Here's the drawing with two shaded views (mm, measured from the low corner). I have some questions. A direction names the side the tool comes from. Round coordinates to 2 decimals unless told otherwise and drop trailing zeros. Return JSON: item names as keys, results as strings. Group by question number.
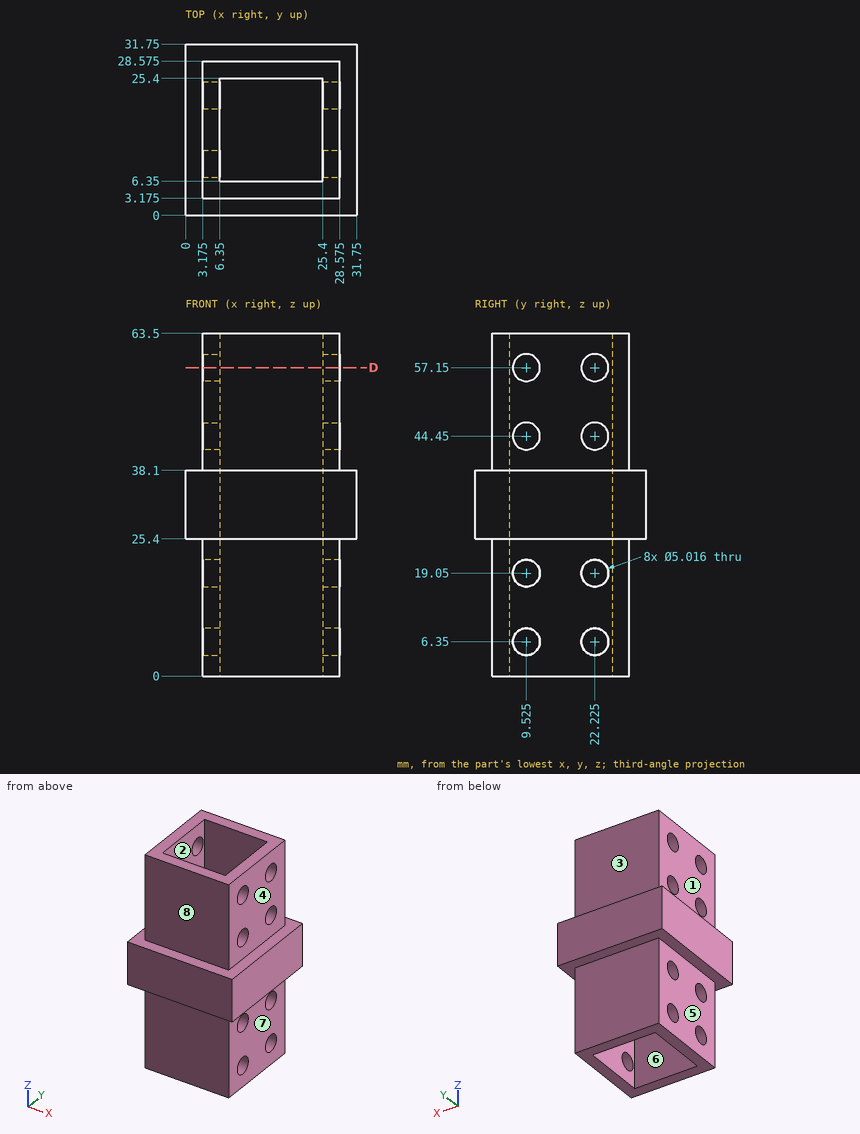
1) We'd pull the mould along X, two halves only. Please class the marked faces 1, 2 and 3: +X half, -X half, draft (parallel to the pull), parting line (faces both ways), or undercut.
2) Will these pins go through, and if not, where does the flat tip stop? pin 1 (1.5 mm diameter, centred on x = 11, z = 18, fed in from -Y) (1 decimal); pin 2 (6 mm diameter, centred on y = 9.525, z = 44.45, fed in from -X) (1 decimal); pin 3 (6.5 mm diameter, centred on y = 22.225, z = 44.45, fed in from +X) (1 decimal).
3) I want a section at D-D, the plane z = 57.15. Give the number of separate pieces and of enclosed holes in the cut face.
4) For the marked faces 4, 5, 6, 7 and 8, which set-ups out of +Z, -Z, +X, -X, +Y, -Y let a thin tool reach every point of the face, with its end or its side?
5) If I drill on line 1 along Y through (x, z) = (5.2, 57.15) (1 decimal); line 2 along Y through (x, z) = (5, 44) (1 decimal); line 3 along Y through (x, z) = (18.5, 30), over which ranges is the centre line in solid material (lowest first)? Write a range as from..to.
Outcome:
{
 "1": {"face 1": "-X half", "face 2": "undercut", "face 3": "draft"},
 "2": {"pin 1": "y = 3.2", "pin 2": "x = 3.2", "pin 3": "x = 28.6"},
 "3": {"separate pieces": "4", "enclosed holes": "0"},
 "4": {"face 4": "+Z, +X, +Y, -Y", "face 5": "-Z, -X, +Y, -Y", "face 6": "+Z, -Z", "face 7": "-Z, +X, +Y, -Y", "face 8": "+Z, +X, -X, -Y"},
 "5": {"line 1": "3.2..7, 12..19.7, 24.7..28.6", "line 2": "3.2..7.1, 12..19.8, 24.7..28.6", "line 3": "0..6.35, 25.4..31.75"}
}
